```python
from build123d import *

# Parameters (mm, degrees)
SKETCH1_W           = 200
SKETCH1_H           = 20
BOSS_EXTRUDE1_DEPTH = 1
SKETCH4_W           = 200
SKETCH4_H           = 21
SKETCH4_R           = 2.5
BOSS_EXTRUDE2_DEPTH = 1
SKETCH5_R           = 4
CUT_EXTRUDE1_DEPTH  = 10


with BuildPart() as part:
    # Sketch1 → Boss-Extrude1 (new body)
    with BuildSketch(Plane.XY):
        with Locations((-100, 10)):
            Rectangle(SKETCH1_W, SKETCH1_H)
    extrude(amount=BOSS_EXTRUDE1_DEPTH)

    # Sketch4 → Boss-Extrude2 (add)
    with BuildSketch(Plane(origin=(0, 20, 0), x_dir=(1, 0, 0), z_dir=(0, 1, 0))):
        with Locations((-100, -10.5)):
            Rectangle(SKETCH4_W, SKETCH4_H)
        with Locations(Location((-190, -16, 0), (0, 0, 270))):
            Circle(SKETCH4_R, mode=Mode.SUBTRACT)
        with Locations(Location((-145, -5, 0), (0, 0, 270))):
            Circle(SKETCH4_R, mode=Mode.SUBTRACT)
        with Locations(Location((-100, -16, 0), (0, 0, 270))):
            Circle(SKETCH4_R, mode=Mode.SUBTRACT)
        with Locations(Location((-55, -5, 0), (0, 0, 270))):
            Circle(SKETCH4_R, mode=Mode.SUBTRACT)
        with Locations(Location((-10, -16, 0), (0, 0, 270))):
            Circle(SKETCH4_R, mode=Mode.SUBTRACT)
    extrude(amount=BOSS_EXTRUDE2_DEPTH)

    # Sketch5 → Cut-Extrude1 (cut)
    with BuildSketch(Plane.XY.offset(1)):
        with Locations((-140, 9.372455226)):
            Circle(SKETCH5_R)
        with Locations((-60, 9.372455226)):
            Circle(SKETCH5_R)
    extrude(amount=-CUT_EXTRUDE1_DEPTH, mode=Mode.SUBTRACT)


solid = part.part
```
Build history of the part. All positions in model axes, mm. A direction names the side the tool comes from. Round coordinates to 2 decimals unless told otherwise and drop trailing zeros. Order: outer loops, then holes, each group sorted by start corner. A loop starts at its lowest first (then second) coordinate and runs counter-clockwise, first axis right, second up. Notation, with made-up numbers: (83.25, 35.5) - (103.25, 35.5) arc R20 cw to (103.25, 49.5) - close; hole circle Ø11 at (21, 70). An arc over 180 degrees is marked (long way). Use a Markdown table: item, result.
1) Saw through at C-C on z = 15.5. Write the cut outline in (x, y).
Recorded:
| item | result |
|---|---|
| outline | (-200, 20) - (-192.45, 20) - (-192.45, 21) - (-200, 21) - close; (-187.55, 20) - (-102.45, 20) - (-102.45, 21) - (-187.55, 21) - close; (-97.55, 20) - (-12.45, 20) - (-12.45, 21) - (-97.55, 21) - close; (-7.55, 20) - (0, 20) - (0, 21) - (-7.55, 21) - close |
2) Saw through at B-B on z = 5.5. Write the cut outline in (x, y), and give its area (3 significant figures).
Recorded:
| item | result |
|---|---|
| outline | (-200, 20) - (-147.45, 20) - (-147.45, 21) - (-200, 21) - close; (-142.55, 20) - (-57.45, 20) - (-57.45, 21) - (-142.55, 21) - close; (-52.55, 20) - (0, 20) - (0, 21) - (-52.55, 21) - close |
| area | 190 mm² |
3) Saw through at D-D on x = -190. Write the cut outline in (y, z), and give its area (3 significant figures).
Recorded:
| item | result |
|---|---|
| outline | (0, 0) - (21, 0) - (21, 13.5) - (20, 13.5) - (20, 1) - (0, 1) - close; (20, 18.5) - (21, 18.5) - (21, 21) - (20, 21) - close |
| area | 36.0 mm² |
4) Wall check: L1, parallel to X at y = 20.45, z = 16; L2, parallel to X at y = 20.6, z = 5; L3, parallel to Y at x = -140, z = 0.55. Give the ranges that are in metal, low to high.
Recorded:
| item | result |
|---|---|
| L1 | x = -200 to -192.5, -187.5 to -102.5, -97.5 to -12.5, -7.5 to 0 |
| L2 | x = -200 to -147.5, -142.5 to -57.5, -52.5 to 0 |
| L3 | y = 0 to 5.37, 13.37 to 21 |
5) Pull direction X, two halves, no side cores. Call faces 1 (the face through (-200, 20.6, 5.9)), 2 (the face through (-101, 20, 11)), 3 (the face through (-136.185, 10.574, 0.507)), 4 (the face through (-97.52, 20.49, 15.67)): pulls with the +X half, pulls with the -X half, needs draft (parallel to the pull), parting line crosses it, or undercut.
Recorded:
| item | result |
|---|---|
| face 1 | pulls with the -X half |
| face 2 | needs draft |
| face 3 | undercut |
| face 4 | undercut |
6) Tool access for faces 5 (the face through (-101, 10, 0)), 6 (the face through (-101, 10, 1)): list every direction of +Z, -Z, +X, -X, +Y, -Y with a clear straight run to the whole face (end or side of a thin tool).
Recorded:
| item | result |
|---|---|
| face 5 | -Z, +X, -X, +Y, -Y |
| face 6 | +Z, +X, -X, -Y |
7) Saw through at A-A on x = -140. Write the cut outline in (y, z).
Recorded:
| item | result |
|---|---|
| outline | (0, 0) - (5.37, 0) - (5.37, 1) - (0, 1) - close; (13.37, 0) - (21, 0) - (21, 21) - (20, 21) - (20, 1) - (13.37, 1) - close |
8) Flat gauge pins, fed straight in: pin 1 Ø5 at (x, y) = (-89, 7) entering from +Z; pin 2 Ø10 at (x, z) = (-124, 8.5) entering from -Y. Where does each tip first touch, or does it go through?
Recorded:
| item | result |
|---|---|
| pin 1 | stops at z = 1 |
| pin 2 | stops at y = 20 |
